Build history of the part. All positions in model axes, mm. Give positions to 0.01 mm unless a question says otherwise; leave off trailing zeros. Write each loop counter-clockwise with the first axis right and the second up, starting at its lowest first coordinate (ties: lowest second). Pieces come first, ordered by that corner, then holes. Notation, with made-up numbers: M 32.25,23 L 71.25,23 A26 ccw 71.25,52 Z; hole C -30,49 d2. An arc over 180 degrees is marked long. Return JSON: item names as keys, results as strings. Group by question number.
Q1. Band-saw the part on C-C, the plane z = -68. Give the cut face in (x, y).
Q2. Band-saw the part on D-D, the plane x = -73. Give the cut face in (y, z), then the cut area to 3 significant figures.
Q3. Band-saw the part on B-B, the plane x = 34. Give the cut face in (y, z).
Q4. Flat gauge pins, fed straight in: pin 1 Ø3 at (y, z) = (4.5, -87) entering from +X; pin 2 Ø1 at (y, z) = (5, -47.5) entering from +X; pin 3 Ø1.5 at (x, y) = (-43, 2) entering from -Z. Where does each tip first touch, or does it go through?
Q5. Wall check: probe 1 along X at (y, z) = (4.5, 0); probe 2 along Y at (x, z) = (0, 54.5); probe 3 along X at (y, z) = (4.5, -92). Give the ranges that are in metal, low to high.
Q6. Band-saw the part on A-A, the plane z = 0. Give the cut face in (x, y).
from build123d import *

# Parameters (mm, degrees)
SKETCH1_R           = 50.8
BOSS_EXTRUDE1_DEPTH = 6.35
SKETCH2_R           = 1.5875
CUT_EXTRUDE1_DEPTH  = 12.724811
CIRPATTERN1_COUNT   = 3


with BuildPart() as part:
    # Sketch1 → Boss-Extrude1 (new body)
    with BuildSketch(Plane(origin=(0, 0, 0), x_dir=(1, 0, 0), z_dir=(0, 1, 0))):
        with BuildLine():
            Line((-19.05, 112.701319868), (-19.05, 60.57513929))
            ThreePointArc((-19.05, 60.57513929), (-54.99261314, 31.75), (-61.984609463, -13.789785703))
            Line((-61.984609463, -13.789785703), (-107.127206046, -39.852875992))
            Line((-107.127206046, -39.852875992), (-118.265853064, -46.283776846))
            ThreePointArc((-118.265853064, -46.283776846), (-109.985226281, -63.5), (-99.215853064, -79.27934473))
            Line((-99.215853064, -79.27934473), (-88.077206046, -72.848443876))
            Line((-88.077206046, -72.848443876), (-42.934609463, -46.785353587))
            ThreePointArc((-42.934609463, -46.785353587), (0, -63.5), (42.934609463, -46.785353587))
            Line((42.934609463, -46.785353587), (88.077206046, -72.848443876))
            Line((88.077206046, -72.848443876), (99.215853064, -79.27934473))
            ThreePointArc((99.215853064, -79.27934473), (109.985226281, -63.5), (118.265853064, -46.283776846))
            Line((118.265853064, -46.283776846), (107.127206046, -39.852875992))
            Line((107.127206046, -39.852875992), (61.984609463, -13.789785703))
            ThreePointArc((61.984609463, -13.789785703), (54.99261314, 31.75), (19.05, 60.57513929))
            Line((19.05, 60.57513929), (19.05, 112.701319868))
            Line((19.05, 112.701319868), (19.05, 125.563121576))
            ThreePointArc((19.05, 125.563121576), (0, 127), (-19.05, 125.563121576))
            Line((-19.05, 125.563121576), (-19.05, 112.701319868))
        make_face()
        with Locations(Location((0, 0, 0), (0, 0, 270))):  # turned: the seam where the file's is
            Circle(SKETCH1_R, mode=Mode.SUBTRACT)
    extrude(amount=BOSS_EXTRUDE1_DEPTH)

    # Sketch2 → Cut-Extrude1 (cut)
    with BuildSketch(Plane.XY.offset(63.5)):
        with Locations((0, 3.175)):
            Circle(SKETCH2_R)
    cut_extrude1 = extrude(amount=-CUT_EXTRUDE1_DEPTH, mode=Mode.SUBTRACT)

    # CirPattern1: Cut-Extrude1 ×3 about axis
    cirpattern1_axis = Axis((0, 0, 0), (0, -1, 0))
    for i in range(1, CIRPATTERN1_COUNT):
        add(cut_extrude1.rotate(cirpattern1_axis, i * 360 / CIRPATTERN1_COUNT), mode=Mode.SUBTRACT)


solid = part.part
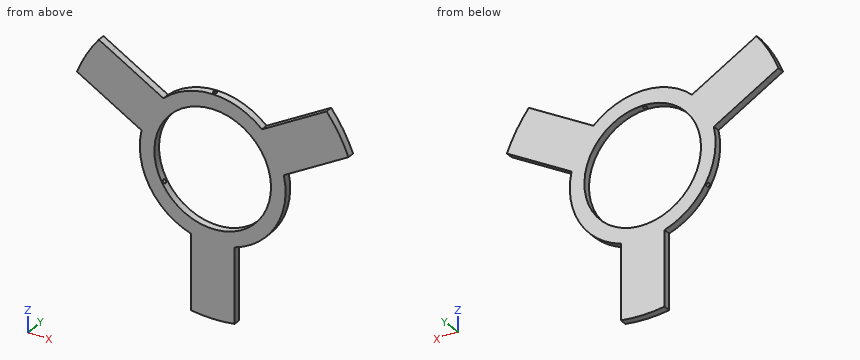
From the geometry:
{
 "1": {"outline": "M -19.05,0 L 19.05,0 L 19.05,6.35 L -19.05,6.35 Z"},
 "2": {"outline": "M 0,20.15 L 6.35,20.15 L 6.35,64.14 L 0,64.14 Z", "area": "279 mm^2"},
 "3": {"outline": "M 0,-53.63 L 6.35,-53.63 L 6.35,-37.74 L 0,-37.74 Z; M 0,37.74 L 6.35,37.74 L 6.35,53.63 L 0,53.63 Z"},
 "4": {"pin 1": "stops at x = 19.05", "pin 2": "stops at x = 42.7", "pin 3": "stops at z = -47.4"},
 "5": {"probe 1": "x = -63.5 to -50.8, 50.8 to 63.5", "probe 2": "y = 0 to 1.59, 4.76 to 6.35", "probe 3": "x = -19.05 to 19.05"},
 "6": {"outline": "M -63.5,0 L -50.8,0 L -50.8,6.35 L -63.5,6.35 Z; M 50.8,0 L 63.5,0 L 63.5,6.35 L 50.8,6.35 Z"}
}
